Work out the finished part from the listing and answer in its coordinate system (mm). A direction names the side the tool comes from. Round coordinates to 2 decimals unless told otherwise and drop trailing zeros. Order: outer loops, then holes, each group sorted by start corner. A loop starts at its lowest first (then second) coordinate and runs counter-clockwise, first axis right, second up. Notation, with made-up numbers: (64.25, 53) - (87.25, 53) arc R21 cw to (87.25, 66) - close; hole circle Ø2 at (14.25, 10.5). An arc over 180 degrees is marked (long way). Answer in a Markdown table with one row per item.
from build123d import *

# Parameters (mm, degrees)
SKETCH_1_R          = 14.5
EXTRUDE_1_DEPTH     = 2
EXTRUDE_START       = 2
EXTRUDE_2_DEPTH     = 0.8
SKETCH_1_4_R        = 1.75
CUT_EXTRUDE_1_DEPTH = 2.8


with BuildPart() as part:
    # Эскиз1 → Бобышка-Вытянуть1 (new body)
    with BuildSketch(Plane.XY):
        Circle(SKETCH_1_R)
    extrude(amount=EXTRUDE_1_DEPTH)

    # Эскиз1<3> → Бобышка-Вытянуть2 (add)
    with BuildSketch(Plane.XY.offset(EXTRUDE_START)):
        with BuildLine():
            Line((-2.5, -4.038873605), (-2.5, -9.25))
            ThreePointArc((-2.5, -9.25), (0, -11.75), (2.5, -9.25))
            Line((2.5, -9.25), (2.5, -4.038873605))
            ThreePointArc((2.5, -4.038873605), (0, 4.75), (-2.5, -4.038873605))
        make_face()
    extrude(amount=EXTRUDE_2_DEPTH)

    # Эскиз1<4> → Вырез-Вытянуть1 (cut)
    with BuildSketch(Plane.XY):
        Circle(SKETCH_1_4_R)
    extrude(amount=CUT_EXTRUDE_1_DEPTH, mode=Mode.SUBTRACT)


solid = part.part
1) Find section B-B, the plane y = 0. Give the vertices of the cut face in (x, z), then the cut area to 3 significant figures.
Filled in:
| item | result |
|---|---|
| outline | (-14.5, 0) - (-1.75, 0) - (-1.75, 2.8) - (-4.75, 2.8) - (-4.75, 2) - (-14.5, 2) - close; (1.75, 0) - (14.5, 0) - (14.5, 2) - (4.75, 2) - (4.75, 2.8) - (1.75, 2.8) - close |
| area | 55.8 mm^2 |
2) Find section D-D, the plane y = 3. Give the vertices of the cut face in (x, z).
Filled in:
| item | result |
|---|---|
| outline | (-14.19, 0) - (14.19, 0) - (14.19, 2) - (3.68, 2) - (3.68, 2.8) - (-3.68, 2.8) - (-3.68, 2) - (-14.19, 2) - close |
3) Find the intervals of material crossed by probe 1 along Y at (x, z) = (0, 0.7); probe 2 along Z at (x, y) = (8.5, -5.25); probe 3 along X at (y, z) = (6, 1.7), in increasing order. Write a range as from..to.
Filled in:
| item | result |
|---|---|
| probe 1 | y = -14.5..-1.75, 1.75..14.5 |
| probe 2 | z = 0..2 |
| probe 3 | x = -13.2..13.2 |
4) Each of these flat-tipped pins is pushed along its axis until it touches: pin 1 (1 mm diameter, centred on x = 4, z = 1.5, fed in from -Y); pin 2 (0.9 mm diameter, centred on y = -5.5, z = 2.5, fed in from +X); pin 3 (1.5 mm diameter, centred on x = -7, z = 1.5, fed in from +Y). Where does it stop, or does it pass through?
Filled in:
| item | result |
|---|---|
| pin 1 | stops at y = -14.07 |
| pin 2 | stops at x = 2.5 |
| pin 3 | stops at y = 13.08 |
5) The mould has two halves that part along X. Classify faces 4 (the face through (3, 0, 0)), 5 (the face through (0.172, 4.747, 2.394)), 6 (the face through (1.617, -0.67, 1.38)): released by +X, released by -X, zero draft, split by the parting line, or undercut.
Filled in:
| item | result |
|---|---|
| face 4 | zero draft |
| face 5 | split by the parting line |
| face 6 | undercut |
6) Find section C-C, the plane z = 2.35. Give the vertices of the cut face in (x, y).
Filled in:
| item | result |
|---|---|
| outline | (-2.5, -9.25) arc R2.5 ccw to (2.5, -9.25) - (2.5, -4.04) arc R4.75 ccw (long way) to (-2.5, -4.04) - close; hole circle Ø3.5 at (0, 0) |
7) Which of the six approach directions +Z, -Z, +X, -X, +Y, -Y give full straight-line access (tool end or side, diameter ignored) to faces 1 (the face through (6, 0, 2)), 2 (the face through (6.691, -12.864, 0.986)), 3 (the face through (-0.05, -11.75, 2.39))?
Filled in:
| item | result |
|---|---|
| face 1 | +Z |
| face 2 | +Z, -Z |
| face 3 | +Z, -Y |
8) Find section A-A, the plane x = 0. Give the vertices of the cut face in (y, z), then the cut area to 3 significant figures.
Filled in:
| item | result |
|---|---|
| outline | (-14.5, 0) - (-1.75, 0) - (-1.75, 2.8) - (-11.75, 2.8) - (-11.75, 2) - (-14.5, 2) - close; (1.75, 0) - (14.5, 0) - (14.5, 2) - (4.75, 2) - (4.75, 2.8) - (1.75, 2.8) - close |
| area | 61.4 mm^2 |
